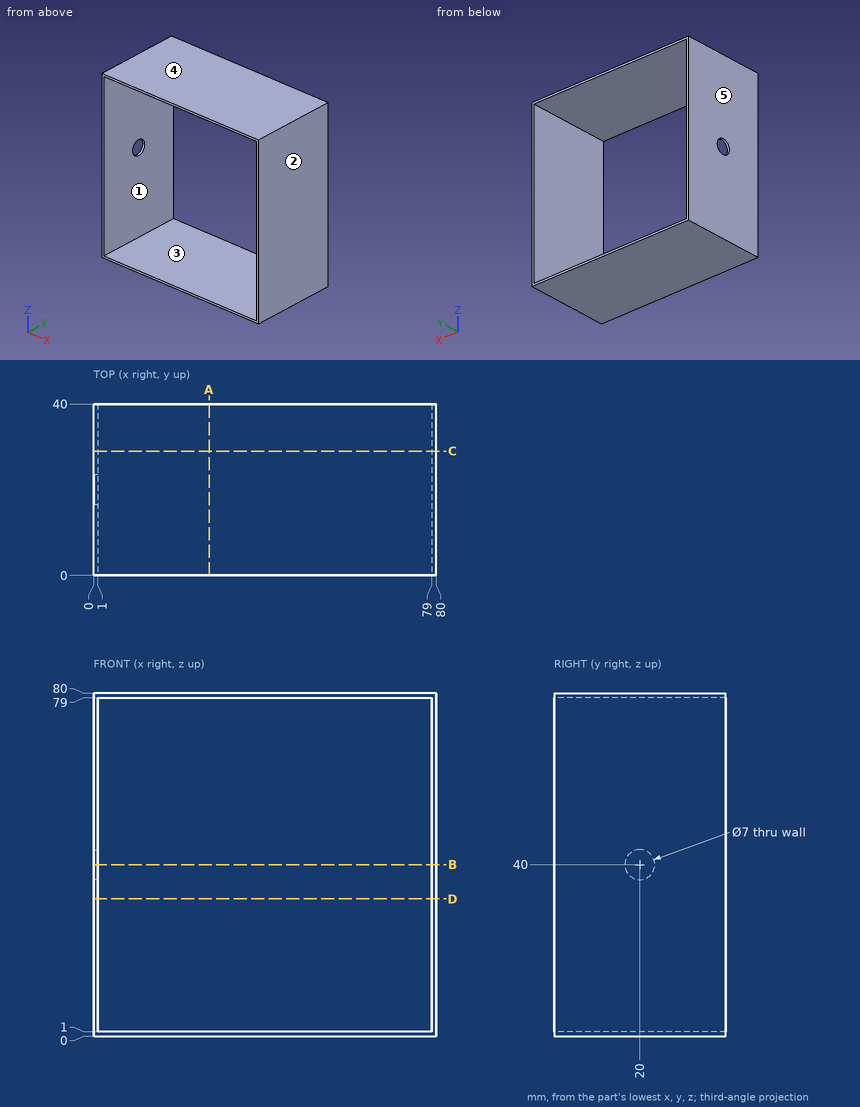
Drawing for the job (mm, zero at the part's lowest x, y, z). A direction names the side the tool comes from. Give positions to 0.01 mm unless a question says otherwise; leave off trailing zeros. Loops run counter-clockwise (first coordinate to the right, second up) from the corner with the lowest first, then second, coordinate; pieces in that order, holes last.
Item 1: Slice it at D-D (z = 32). Write the cut outline in (x, y), plus the area to 3 significant figures.
Check values:
outline: (0, 0) - (1, 0) - (1, 40) - (0, 40) - close; (79, 0) - (80, 0) - (80, 40) - (79, 40) - close
area: 80.0 mm2
Item 2: Drill centre lines: line 1 along Z through (x, y) = (75.5, 18.5); line 2 along Z through (x, y) = (0.7, 20). Where is each one in solid material? Low to high.
Check values:
line 1: z = 0 to 1, 79 to 80
line 2: z = 0 to 36.5, 43.5 to 80
Item 3: Mould opens along Z. For the marked faces 3, 4 and 5 say: +Z half, -Z half, draft (parallel to the pull), parting line (faces both ways), or undercut.
Check values:
face 3: undercut
face 4: +Z half
face 5: draft
Item 4: Slice it at A-A (x = 27). Write the cut outline in (y, z), plus the area to 3 significant figures.
Check values:
outline: (0, 0) - (40, 0) - (40, 1) - (0, 1) - close; (0, 79) - (40, 79) - (40, 80) - (0, 80) - close
area: 80.0 mm2
Item 5: Drop flat-ended pins along their axis: P1, Ø1.5, axis at y = 6, z = 13.5, coming from the -X side; P2, Ø6.5, axis at y = 20, z = 40, coming from the -X side. Give the stop position or say it passes through.
Check values:
P1: stops at x = 0
P2: stops at x = 79
Item 6: Which spindle directions (+Z, -Z, +X, -X, +Y, -Y) get a long thin tool onto all of the face, cutting with end or side? Do the marked faces 1 and 2. Say none if no direction does.
Check values:
face 1: +Y, -Y
face 2: +Z, -Z, +X, +Y, -Y
Item 7: Slice it at B-B (z = 40). Write the cut outline in (x, y).
Check values:
outline: (0, 0) - (1, 0) - (1, 16.5) - (0, 16.5) - close; (0, 23.5) - (1, 23.5) - (1, 40) - (0, 40) - close; (79, 0) - (80, 0) - (80, 40) - (79, 40) - close
Item 8: Slice it at C-C (y = 29). Write the cut outline in (x, z), plus the area to 3 significant figures.
Check values:
outline: (0, 0) - (80, 0) - (80, 80) - (0, 80) - close; hole (1, 1) - (79, 1) - (79, 79) - (1, 79) - close
area: 316 mm2
